For this review, take the finished solid that the model builds, in its own axes (mm). A direction names the side the tool comes from. Coordinates: 2 decimals unless noted, no trailing zeros. Loops run counter-clockwise (first coordinate to the right, second up) from the corner with the lowest first, then second, coordinate; pieces in that order, holes last.
Autodesk Inventor part; units mm, degrees
ref_plane "YZ Plane" through (0, 0, 0) normal (1, 0, 0) x (0, 1, 0)
ref_plane "XZ Plane" through (0, 0, 0) normal (0, 1, 0) x (-1, 0, 0)
ref_plane "XY Plane" through (0, 0, 0) normal (0, 0, 1) x (1, 0, 0)
sketch "Sketch1" plane through (0, 0, 0) normal (0, 0, 1) x (1, 0, 0)
  line L0 (0, 0) -> (12, 0)
  line L1 (12, 0) -> (12, 10)
  line L2 (12, 10) -> (0, 10)
  line L3 (0, 10) -> (0, 0)
  line L4 (6, 10) -> (6, 0) construction
  line L5 (1.5, 5) -> (10.5, 5) construction
  circle A0 centre (1.5, 5) radius 0.8
  circle A1 centre (10.5, 5) radius 0.8
  circle A2 centre (6, 5) radius 1.5
  dimension "d0" = 10
  dimension "d1" = 12
  dimension "d2" = 9
  dimension "d3" = 1.6
  dimension "d4" = 3
extrude "Extrusion1" add sketch "Sketch1" against normal blind 9 contours L3 L2 L1 L0 | A0 | A1 | A2
extrude "Extrusion2" cut sketch "Sketch1" against normal through all contours A0 | A1
extrude "Extrusion3" add sketch "Sketch1" along normal blind 10 contours A2
sketch "Sketch2" plane through (6, 5, 10) normal (0, 0, 1) x (1, 0, 0)
  circle A0 centre (0, 0) radius 1.5
  circle A1 centre (0, 0) radius 1.5
  line L0 (-1.118, 1) -> (1.118, 1)
  point P0 (-6, -5)
  point P1 (-1.118, 1)
  point P2 (1.118, 1)
  dimension "d11" = 1
extrude "Extrusion4" cut sketch "Sketch2" against normal blind 9.8 contours L0 A0 picked at (-0.0599, 1.1631)
sketch "Sketch3" plane through (0, 0, -9) normal (0, 0, -1) x (-1, 0, 0)
  circle A0 centre (-6, 5) radius 1.5
  circle A1 centre (-6, 5) radius 6
  circle A2 centre (-10.5, 5) radius 0.8
  circle A3 centre (-1.5, 5) radius 0.8
  line L0 (-12, 0) -> (0, 0)
  line L1 (0, 0) -> (0, 10)
  line L2 (0, 10) -> (-12, 10)
  line L3 (-12, 10) -> (-12, 0)
  point P0 (-2.6834, 10)
  point P1 (-9.3166, 10)
  point P2 (-9.3166, 0)
  point P3 (-2.6834, 0)
extrude "Extrusion5" add sketch "Sketch3" along normal blind 15.4 contours A0 | A1 L0 L2 | A2 | A3
sketch "Sketch4" plane through (0, 0, -24.4) normal (0, 0, -1) x (-1, 0, 0)
  arc A0 (-2.6834, 0) -> (-2.6834, 10) centre (-6, 5) ccw
  circle A1 centre (-6, 5) radius 2.5
  point P0 (0, 0)
  dimension "d16" = 5
extrude "Extrusion6" add sketch "Sketch4" along normal blind 0.8
fillet "Fillet1" radius 0.5 4 edges at (12, 10, -4.5) (0, 10, -4.5) (12, 0, -4.5) (0, 0, -4.5)
properties part number "n20"
Q1. Consider section C-C (y = 8.25). State the section outline as (x, z) points, then the cut area to 3 significant figures.
Q2. Consider section B-B (x = 6). State the section outline as (y, z) points.
Q3. Consider section D-D (z = -11.5). State the section outline as (x, y) points.
Q4. The part is to be moulded in two halves that separate along Y. For faces 1 (the face through (11, 5, -9)), 2 (the face through (4.6, 6.2, 0)), 3 (the face through (6, 0, -9)), say which applies: +Y half, -Y half, draft (parallel to the pull), parting line (faces both ways), or undercut.
Q5. For pin 1 Ø1.5 at (x, y) = (4.5, 7.5) entering from +Z; pin 2 Ø2 at (x, y) = (2, 8) entering from -Z; pin 3 Ø1.5 at (x, z) = (6, 5) entering from -Y, all flat-tipped, find the tip position at first contact; note any pin that passes through.
Q6. Wall thickness on probe 1 along Y at (x, z) = (1.5, -5.75); probe 2 along Z at (x, y) = (8.5, 0.5); probe 3 along X at (y, z) = (4, 4): over which ranges is each line inside the solid? List them lowest first.
Q7. Machinability: for faces 4 (the face through (2, 5, -9)), 5 (the face through (0, 5, -17)), 6 (the face through (3.615, 4.249, -24.794)), 7 (the face through (11, 1, -9)), 8 (the face through (11, 9, -9)), which of the approach directions +Z, -Z, +X, -X, +Y, -Y give a long, thin tool a straight path to every point of the face, cutting with its end or side? Answer none if there is none.
Q8. Consider section A-A (z = -4.5). State the section outline as (x, y) points.
Model answer:
1. outline: (0, -9) - (0.96, -9) - (0.96, -24.4) - (11.04, -24.4) - (11.04, -9) - (12, -9) - (12, 0) - (0, 0) - close
1. area: 263 mm2
2. outline: (0, -24.4) - (2.5, -24.4) - (2.5, -25.2) - (7.5, -25.2) - (7.5, -24.4) - (10, -24.4) - (10, 0) - (6.5, 0) - (6.5, 0.2) - (6, 0.2) - (6, 10) - (3.5, 10) - (3.5, 0) - (0, 0) - close
3. outline: (2.68, 0) - (9.32, 0) arc R6 ccw to (9.32, 10) - (2.68, 10) arc R6 ccw to start
4. face 1: undercut
4. face 2: draft
4. face 3: -Y half
5. pin 1: stops at z = 0
5. pin 2: stops at z = -24.4
5. pin 3: stops at y = 3.5
6. probe 1: y = 0 to 4.2, 5.8 to 10
6. probe 2: z = -24.4 to 0
6. probe 3: x = 4.88 to 7.12
7. face 4: +Z
7. face 5: -Z, -X
7. face 6: -Z
7. face 7: -Z, +X, -Y
7. face 8: -Z, +X, +Y
8. outline: (0, 0.5) arc R0.5 ccw to (0.5, 0) - (11.5, 0) arc R0.5 ccw to (12, 0.5) - (12, 9.5) arc R0.5 ccw to (11.5, 10) - (0.5, 10) arc R0.5 ccw to (0, 9.5) - close; hole circle Ø1.6 at (1.5, 5); hole circle Ø1.6 at (10.5, 5)
